Read the model definition and answer for the solid it produces. Units are mm, in the model's axes. Round coordinates to 2 decimals unless told otherwise and drop trailing zeros. Loops run counter-clockwise (first coordinate to the right, second up) from the corner with the lowest first, then second, coordinate; pieces in that order, holes last. Notation, with made-up numbers: M 34,-12.5 L 42,-12.5 A19 cw 42,4.5 Z; hole C 56.5,69 d2. An arc over 180 degrees is marked long. Write each question's results on one line, items separated by ' | '.
from build123d import *

# Parameters (mm, degrees)
SKETCH1_R           = 2.15
SKETCH1_R_2         = 4.953
SKETCH1_W           = 25.4
SKETCH1_H           = 3.175
BOSS_EXTRUDE1_DEPTH = 1.5875


with BuildPart() as part:
    # Sketch1 → Boss-Extrude1 (new body, symmetric)
    with BuildSketch(Plane(origin=(0, 0, 0), x_dir=(1, 0, 0), z_dir=(0, 1, 0))):
        Polygon((-152.4, 12.7), (-152.4, -88.9), (-114.3, -88.9), (-88.9, -88.9), (-63.5, -88.9), (-38.1, -88.9), (-12.7, -88.9), (12.7, -88.9), (38.1, -88.9), (63.5, -88.9), (88.9, -88.9), (114.3, -88.9), (152.4, -88.9), (152.4, 12.7), (149.225, 12.7), (149.225, -12.7), (146.05, -12.7), (146.05, 88.9), (-146.05, 88.9), (-146.05, -12.7), (-149.225, -12.7), (-149.225, 12.7), align=None)
        with Locations((-6.35, 81.8322)):
            Circle(SKETCH1_R, mode=Mode.SUBTRACT)
        with Locations((25.4, 63.5)):
            Circle(SKETCH1_R_2, mode=Mode.SUBTRACT)
        with Locations((-101.6, -90.4875)):
            Rectangle(SKETCH1_W, SKETCH1_H)
        with Locations((-50.8, -90.4875)):
            Rectangle(SKETCH1_W, SKETCH1_H)
        with Locations((0, -90.4875)):
            Rectangle(SKETCH1_W, SKETCH1_H)
        with Locations((50.8, -90.4875)):
            Rectangle(SKETCH1_W, SKETCH1_H)
        with Locations((101.6, -90.4875)):
            Rectangle(SKETCH1_W, SKETCH1_H)
    extrude(amount=BOSS_EXTRUDE1_DEPTH, both=True)


solid = part.part
Item 1: The part is cut by section A-A (z = -63.5). Determine the outline of the cut face in (x, y).
Outcome:
outline: M -146.05,-1.59 L 20.45,-1.59 L 20.45,1.59 L -146.05,1.59 Z; M 30.35,-1.59 L 146.05,-1.59 L 146.05,1.59 L 30.35,1.59 Z
Item 2: Straight lines are drawn through the part: line 1 (X direction, y = 0.1, z = -5.5) (3 decimals); line 2 (Z direction, x = -6.35, y = -0.3) (3 decimals); line 3 (Z direction, x = 25.4, y = -0.25). For each, find the intervals that lie inside material, in ascending order.
Outcome:
line 1: x = -152.4 to -149.225, -146.05 to 146.05, 149.225 to 152.4 | line 2: z = -88.9 to -83.982, -79.682 to 92.075 | line 3: z = -88.9 to -68.45, -58.55 to 88.9
Item 3: The mould has two halves that part along Z. Classify faces 1 (the face through (24.326, -0.022, -58.665)), 2 (the face through (-2, 1.588, 0)): pulls with the +Z half, pulls with the -Z half, needs draft (parallel to the pull), parting line crosses it, or undercut.
Outcome:
face 1: undercut | face 2: needs draft
Item 4: The part is cut by section D-D (z = -16.5). Determine the outline of the cut face in (x, y).
Outcome:
outline: M -146.05,-1.59 L 146.05,-1.59 L 146.05,1.59 L -146.05,1.59 Z
Item 5: Flat-ended cylindrical pins translate along their axes: pin 1 (5.5 mm diameter, centred on x = -6.35, z = -81.83, fed in from -Y); pin 2 (1 mm diameter, centred on x = 151, y = 0.5, fed in from -Z); pin 3 (1.6 mm diameter, centred on y = -0.5, z = 90.5, fed in from +X); pin 4 (1 mm diameter, centred on y = -0.5, z = 90, fed in from -X). Find the tip coordinate at first contact, or state that the pin passes through.
Outcome:
pin 1: stops at y = -1.59 | pin 2: stops at z = -12.7 | pin 3: stops at x = 114.3 | pin 4: stops at x = -114.3
Item 6: The part is cut by section B-B (x = 25.4). Determine the outline of the cut face in (y, z).
Outcome:
outline: M -1.59,-88.9 L 1.59,-88.9 L 1.59,-68.45 L -1.59,-68.45 Z; M -1.59,-58.55 L 1.59,-58.55 L 1.59,88.9 L -1.59,88.9 Z
Item 7: The part is cut by section C-C (y = 0.95). State how many separate pieces and enclosed holes the cut face has, plus the area to 3 significant figures.
Outcome:
separate pieces: 1 | enclosed holes: 2 | area: 53,400 mm2
